Autodesk Inventor part; units mm, degrees
ref_plane "YZ Plane" through (0, 0, 0) normal (1, 0, 0) x (0, 1, 0)
ref_plane "XZ Plane" through (0, 0, 0) normal (0, 1, 0) x (-1, 0, 0)
ref_plane "XY Plane" through (0, 0, 0) normal (0, 0, 1) x (1, 0, 0)
sketch "Szkic1" plane through (0, 0, 0) normal (0, 0, 1) x (1, 0, 0)
  line L0 (-6.3643, 3.3741) -> (43.6357, 3.3741)
  line L1 (43.6357, 3.3741) -> (43.6357, -16.6259)
  line L2 (43.6357, -16.6259) -> (-6.3643, -16.6259)
  line L3 (-6.3643, -16.6259) -> (-6.3643, 3.3741)
  point P0 (0, 0)
  dimension "d0" = 50
  dimension "d1" = 20
extrude "Wyciągnięcie proste1" add sketch "Szkic1" along normal blind 20
sketch "Szkic2" plane through (0, 0, 20) normal (0, 0, 1) x (1, 0, 0)
  line L0 (43.6357, 3.3741) -> (-6.3643, 3.3741)
  line L1 (-6.3643, 3.3741) -> (-6.3643, -16.6259)
  line L2 (-6.3643, -16.6259) -> (43.6357, -16.6259)
  line L3 (43.6357, -16.6259) -> (43.6357, 3.3741)
  line L4 (-3.3643, 0.3741) -> (40.6357, 0.3741)
  line L5 (40.6357, -13.6259) -> (-3.3643, -13.6259)
  line L6 (-3.3643, -13.6259) -> (-3.3643, -10.6259)
  line L7 (-3.3643, -2.6259) -> (-3.3643, 0.3741)
  line L8 (-6.3643, -2.6259) -> (-3.3643, -2.6259)
  line L9 (40.6357, -2.6259) -> (43.6357, -2.6259)
  line L10 (-6.3643, -10.6259) -> (-3.3643, -10.6259)
  line L11 (40.6357, -10.6259) -> (43.6357, -10.6259)
  line L12 (40.6357, 0.3741) -> (40.6357, -2.6259)
  line L13 (40.6357, -10.6259) -> (40.6357, -13.6259)
  point P0 (0, 0)
  dimension "d4" = 3
  dimension "d7" = 6
  dimension "d8" = 6
  dimension "d9" = 6
  dimension "d10" = 6
  dimension "d11" = 3
  dimension "d12" = 3
  dimension "d13" = 3
  dimension "d14" = 3
extrude "Wyciągnięcie proste2" add sketch "Szkic2" along normal blind 5 contours L3 L9 L12 L4 L7 L8 L1 L0 | L3 L2 L1 L10 L6 L5 L13 L11
sketch "Szkic3" plane through (0, 0, 25) normal (0, 0, 1) x (1, 0, 0)
  line L0 (-6.3643, -16.6259) -> (43.6357, -16.6259)
  line L1 (43.6357, -16.6259) -> (43.6357, -10.6259)
  line L2 (43.6357, -10.6259) -> (40.6357, -10.6259)
  line L3 (40.6357, -10.6259) -> (40.6357, -13.6259)
  line L4 (40.6357, -13.6259) -> (-3.3643, -13.6259)
  line L5 (-3.3643, -13.6259) -> (-3.3643, -10.6259)
  line L6 (-3.3643, -10.6259) -> (-6.3643, -10.6259)
  line L7 (-6.3643, -10.6259) -> (-6.3643, -16.6259)
  line L8 (-6.3643, -16.6259) -> (43.6357, -16.6259)
  line L9 (-5.3643, -16.6259) -> (-3.3643, -16.6259)
  line L10 (-5.3643, -16.6259) -> (-4.3643, -15.6259)
  line L11 (-4.3643, -15.6259) -> (-3.3643, -16.6259)
  point P0 (0, 0)
  dimension "d17" = 2
  dimension "d18" = 1
  dimension "d19" = 1
extrude "Wyciągnięcie proste3" cut sketch "Szkic3" against normal through all contours L10 L11 L0
pattern_linear "Szyk prostokątny1" count 24 spacing 2 along (1, 0, 0) of "Wyciągnięcie proste3"
sketch "Szkic4" plane through (0, 0, 0) normal (0, 0, -1) x (-1, 0, 0)
  line L0 (-42.6357, -16.6259) -> (-41.6357, -15.6259)
  line L1 (-41.6357, -15.6259) -> (-40.6357, -16.6259)
  line L2 (-40.6357, -16.6259) -> (-39.6357, -15.6259)
  line L3 (-39.6357, -15.6259) -> (-38.6357, -16.6259)
  line L4 (-38.6357, -16.6259) -> (-37.6357, -15.6259)
  line L5 (-37.6357, -15.6259) -> (-36.6357, -16.6259)
  line L6 (-36.6357, -16.6259) -> (-35.6357, -15.6259)
  line L7 (-35.6357, -15.6259) -> (-34.6357, -16.6259)
  line L8 (-34.6357, -16.6259) -> (-33.6357, -15.6259)
  line L9 (-33.6357, -15.6259) -> (-32.6357, -16.6259)
  line L10 (-32.6357, -16.6259) -> (-31.6357, -15.6259)
  line L11 (-31.6357, -15.6259) -> (-30.6357, -16.6259)
  line L12 (-30.6357, -16.6259) -> (-29.6357, -15.6259)
  line L13 (-29.6357, -15.6259) -> (-28.6357, -16.6259)
  line L14 (-28.6357, -16.6259) -> (-27.6357, -15.6259)
  line L15 (-27.6357, -15.6259) -> (-26.6357, -16.6259)
  line L16 (-26.6357, -16.6259) -> (-25.6357, -15.6259)
  line L17 (-25.6357, -15.6259) -> (-24.6357, -16.6259)
  line L18 (-24.6357, -16.6259) -> (-23.6357, -15.6259)
  line L19 (-23.6357, -15.6259) -> (-22.6357, -16.6259)
  line L20 (-22.6357, -16.6259) -> (-21.6357, -15.6259)
  line L21 (-21.6357, -15.6259) -> (-20.6357, -16.6259)
  line L22 (-20.6357, -16.6259) -> (-19.6357, -15.6259)
  line L23 (-19.6357, -15.6259) -> (-18.6357, -16.6259)
  line L24 (-18.6357, -16.6259) -> (-17.6357, -15.6259)
  line L25 (-17.6357, -15.6259) -> (-16.6357, -16.6259)
  line L26 (-16.6357, -16.6259) -> (-15.6357, -15.6259)
  line L27 (-15.6357, -15.6259) -> (-14.6357, -16.6259)
  line L28 (-14.6357, -16.6259) -> (-13.6357, -15.6259)
  line L29 (-13.6357, -15.6259) -> (-12.6357, -16.6259)
  line L30 (-12.6357, -16.6259) -> (-11.6357, -15.6259)
  line L31 (-11.6357, -15.6259) -> (-10.6357, -16.6259)
  line L32 (-10.6357, -16.6259) -> (-9.6357, -15.6259)
  line L33 (-9.6357, -15.6259) -> (-8.6357, -16.6259)
  line L34 (-8.6357, -16.6259) -> (-7.6357, -15.6259)
  line L35 (-7.6357, -15.6259) -> (-6.6357, -16.6259)
  line L36 (-6.6357, -16.6259) -> (-5.6357, -15.6259)
  line L37 (-5.6357, -15.6259) -> (-4.6357, -16.6259)
  line L38 (-4.6357, -16.6259) -> (-3.6357, -15.6259)
  line L39 (-3.6357, -15.6259) -> (-2.6357, -16.6259)
  line L40 (-2.6357, -16.6259) -> (-1.6357, -15.6259)
  line L41 (-1.6357, -15.6259) -> (-0.6357, -16.6259)
  line L42 (-0.6357, -16.6259) -> (0.3643, -15.6259)
  line L43 (0.3643, -15.6259) -> (1.3643, -16.6259)
  line L44 (1.3643, -16.6259) -> (2.3643, -15.6259)
  line L45 (2.3643, -15.6259) -> (3.3643, -16.6259)
  line L46 (3.3643, -16.6259) -> (4.3643, -15.6259)
  line L47 (4.3643, -15.6259) -> (5.3643, -16.6259)
  line L48 (5.3643, -16.6259) -> (6.3643, -16.6259)
  line L49 (6.3643, -16.6259) -> (6.3643, 3.3741)
  line L50 (6.3643, 3.3741) -> (-43.6357, 3.3741)
  line L51 (-43.6357, 3.3741) -> (-43.6357, -16.6259)
  line L52 (-43.6357, -16.6259) -> (-42.6357, -16.6259)
  circle A0 centre (-18.6357, -18.3259) radius 5
  point P0 (0, 0)
  point P1 (-18.6357, -3.0259)
  dimension "d25" = 25
  dimension "d26" = 6.4
  dimension "d27" = 10
  dimension "d28" = 15.3
  dimension "d29" = 25
extrude "Wyciągnięcie proste4" cut sketch "Szkic4" against normal blind 3.1 contours A0 L28 L27 L26 L25 L24 L23 L22 L21 L20 L19 | L19 L20 L21 L22 L23 L24 L25 L26 L27 L28 A0
hole "Otwór1" at (18.6357, -3.0259, 0) direction (0, 0, 1) diameter 3 end through all
sketch "Szkic5" plane through (0, 0, 20) normal (0, 0, 1) x (1, 0, 0)
  circle A0 centre (18.6357, -3.0259) radius 1.5
  line L0 (-3.3643, -2.6259) -> (-6.3643, -2.6259)
  line L1 (-6.3643, -2.6259) -> (-6.3643, -10.6259)
  line L2 (-6.3643, -10.6259) -> (-3.3643, -10.6259)
  line L3 (-3.3643, -10.6259) -> (-3.3643, -13.6259)
  line L4 (-3.3643, -13.6259) -> (40.6357, -13.6259)
  line L5 (40.6357, -13.6259) -> (40.6357, -10.6259)
  line L6 (40.6357, -10.6259) -> (43.6357, -10.6259)
  line L7 (43.6357, -10.6259) -> (43.6357, -2.6259)
  line L8 (43.6357, -2.6259) -> (40.6357, -2.6259)
  line L9 (40.6357, -2.6259) -> (40.6357, 0.3741)
  line L10 (40.6357, 0.3741) -> (-3.3643, 0.3741)
  line L11 (-3.3643, 0.3741) -> (-3.3643, -2.6259)
  circle A1 centre (18.6357, -3.0259) radius 3.05
  point P0 (0, 0)
  dimension "d39" = 6.1
extrude "Wyciągnięcie proste5" cut sketch "Szkic5" against normal blind 17 contours A1
properties part number "3DP_ABS_Nozzle_Cleaner"
The listing builds one solid part. Answer for the finished solid, in the listing's coordinates (mm). A direction names the side the tool comes from. Round coordinates to 2 decimals unless told otherwise and drop trailing zeros. Use CSV: the item, a comma, the result in double quotes. Start each with the question number.
(1) Consider L1, parallel to Z at x = 19, y = -9.75; L2, parallel to Y at x = 31.5, z = 23; L3, parallel to X at y = -3.75, z = 4.75. Determine where each line is inside the solid, lowest interval first. Write a range as from..to.
(2) Each of these flat-tipped pins is pushed along its axis until it touches: pin 1 (1.5 mm diameter, centred on x = 7.5, z = 6, fed in from -Y); pin 2 (5 mm diameter, centred on x = 21.5, z = 9.5, fed in from -Y); pin 3 (0.9 mm diameter, centred on x = -4.5, z = 22.5, fed in from -Y). Where does it stop, or does it pass through?
(3) Which of the six approach directions +Z, -Z, +X, -X, +Y, -Y give full straight-line access (tool end or side, diameter ignored) to faces 5 (the face through (18, 0.374, 22)), 6 (the face through (19, -15, 3.1)), 7 (the face through (27.13, -16.13, 12.68))?
(4) The mould has two halves that part along Y. Classify faces 1 (the face through (40.636, -1, 22)), 2 (the face through (18, 3.374, 12)), 3 (the face through (-3.364, -12, 22)), 4 (the face through (36.13, -16.12, 12.68)): released by +Y, released by -Y, zero draft, split by the parting line, or undercut.
A:
1,L1,"z = 0..20"
1,L2,"y = -15.76..-13.63, 0.37..3.37"
1,L3,"x = -6.36..15.67, 21.6..43.64"
2,pin 1,"stops at y = -16.51"
2,pin 2,"stops at y = -16.63"
2,pin 3,"stops at y = -16.21"
3,face 5,"+Z"
3,face 6,"-Z, -Y"
3,face 7,"+Z, -Z, -Y"
4,face 1,"undercut"
4,face 2,"released by +Y"
4,face 3,"undercut"
4,face 4,"released by -Y"
